Source: CAD feature listing. Evaluate the final solid. Frame: model axes, mm. A direction names the side the tool comes from. Round coordinates to 2 decimals unless told otherwise and drop trailing zeros. Order: outer loops, then holes, each group sorted by start corner. A loop starts at its lowest first (then second) coordinate and runs counter-clockwise, first axis right, second up. Notation, with made-up numbers: (67.5, 58.25) -> (126.5, 58.25) arc R22 ccw to (126.5, 64.25) -> close; hole circle Ø7 at (34, 50). An arc over 180 degrees is marked (long way). Answer as CSV lines item,"result".
from build123d import *

# Parameters (mm, degrees)
BOSS_EXTRUDE1_DEPTH      = 30
SKETCH2_R                = 4.091242679
BOSS_EXTRUDE2_DEPTH      = 15
SKETCH3_W                = 20
SKETCH3_H                = 12.982921918
BOSS_EXTRUDE3_DEPTH      = 15
BOSS_EXTRUDE5_DEPTH      = 20
BOSS_EXTRUDE5_DEPTH_BACK = 20
SKETCH5_R                = 2.5


with BuildPart() as part:
    # Sketch1 → Boss-Extrude1 (new, symmetric)
    with BuildSketch(Plane.XY):
        with BuildLine():
            Line((-2.5, 25.377155081), (-2.5, 17.320508076))
            ThreePointArc((-2.5, 17.320508076), (0, -17.5), (2.5, 17.320508076))
            Line((2.5, 17.320508076), (2.5, 25.377155081))
            ThreePointArc((2.5, 25.377155081), (0, -25.5), (-2.5, 25.377155081))
        make_face()
    extrude(amount=BOSS_EXTRUDE1_DEPTH, both=True)

    # Sketch2 → Boss-Extrude2 (add, symmetric)
    with BuildSketch(Plane.XY):
        with Locations((6.293533022, 28.211487403)):
            Circle(SKETCH2_R)
        with Locations((-6.293533022, 28.211487403)):
            Circle(SKETCH2_R)
    extrude(amount=BOSS_EXTRUDE2_DEPTH, both=True)

    # Sketch3 → Boss-Extrude3 (add)
    with BuildSketch(Plane.XY):
        with Locations((0, -29.508539041)):
            Rectangle(SKETCH3_W, SKETCH3_H)
    extrude(amount=-BOSS_EXTRUDE3_DEPTH)

    # Sketch5 → Boss-Extrude5 (add, two sides: drawn at the far end of the back side and taken through both)
    with BuildSketch(Plane(origin=(0, 0, 0), x_dir=(0, 0, -1), z_dir=(1, 0, 0)).offset(-BOSS_EXTRUDE5_DEPTH_BACK)):
        with Locations((0, 28.211487403)):
            Circle(SKETCH5_R)
    extrude(amount=BOSS_EXTRUDE5_DEPTH + BOSS_EXTRUDE5_DEPTH_BACK)


solid = part.part
1. Reachability of faces 3 (the cylindrical face through (7.33, 32.17, -0.21)), 4 (the flat face through (2.5, 21, 0)), 5 (the flat face through (10, -30, -7)) from +Z, -Z, +X, -X, +Y, -Y: full face, straight path, thin tool, end or side. Return the list, or none.
Results below:
face 3,"none"
face 4,"+Z, -Z"
face 5,"+Z, -Z, +X, -Y"
2. Section query B-B on x = -12. Return loops of the section in (y, z).
Results below:
outline,"(-22.5, -30) -> (-12.74, -30) -> (-12.74, 30) -> (-22.5, 30) -> close; (12.74, -30) -> (22.5, -30) -> (22.5, 30) -> (12.74, 30) -> close; circle Ø5 at (28.21, 0)"
3. Pin query (flat end, axial travel): pin 1 (9 mm diameter, centred on y = 20, z = -0.5, fed in from +X); pin 2 (4 mm diameter, centred on y = 28, z = -0.5, fed in from +X); pin 3 (1.5 mm diameter, centred on y = 27, z = 0.5, fed in from -X). Return the tip coordinate at first contact, or that it passes through.
Results below:
pin 1,"x = 20.25"
pin 2,"x = 20"
pin 3,"x = -20"
4. Section query D-D on y = 15. Return loops of the section in (x, z), and give its area (3 significant figures).
Results below:
outline,"(-20.62, -30) -> (-9.01, -30) -> (-9.01, 30) -> (-20.62, 30) -> close; (9.01, -30) -> (20.62, -30) -> (20.62, 30) -> (9.01, 30) -> close"
area,"1,390 mm2"
5. Section query A-A on y = 0. Return loops of the section in (x, z).
Results below:
outline,"(-25.5, -30) -> (-17.5, -30) -> (-17.5, 30) -> (-25.5, 30) -> close; (17.5, -30) -> (25.5, -30) -> (25.5, 30) -> (17.5, 30) -> close"
6. Mould query, pull axis Y, two halves, no side actions, for faces 1 (the flat face through (-6, 28, -15)), 2 (the flat face through (-2.5, 21, 0)). Classes: released by +Y, released by -Y, zero draft, split by the parting line, or undercut.
Results below:
face 1,"zero draft"
face 2,"undercut"
7. Line query: L1, parallel to X at y = 0, z = -7.5; L2, parallel to X at y = -14, z = -22.5; L3, parallel to Y at x = -12.5, z = -12. Output: solid intervals per line, ascending. Write a range as [from, to].
Results below:
L1,"[-25.5, -17.5], [17.5, 25.5]"
L2,"[-21.31, -10.5], [10.5, 21.31]"
L3,"[-22.23, -12.25], [12.25, 22.23]"
8. Section query C-C on x = -0.5. Return loops of the section in (y, z).
Results below:
outline,"(-36, -15) -> (-25.5, -15) -> (-25.5, -30) -> (-17.49, -30) -> (-17.49, 30) -> (-25.5, 30) -> (-25.5, 0) -> (-36, 0) -> close; circle Ø5 at (28.21, 0)"
